from build123d import *

# Parameters (mm, degrees)
PAD_DEPTH       = 10
SKETCH001_W     = 15
SKETCH001_H     = 3
PAD001_DEPTH    = 44
SKETCH002_R     = 14
SKETCH002_R_2   = 1.7
POCKET_DEPTH    = 6.001
SKETCH003_R     = 1.2
POCKET001_DEPTH = 5
POCKET002_DEPTH = 2.5


with BuildPart() as part:
    # Sketch → Pad (new body)
    with BuildSketch(Plane.XZ):
        with BuildLine():
            Line((0, 0), (24, 0))
            ThreePointArc((24, 0), (24.707107, 0.292893), (25, 1))
            Line((25, 1), (25, 2))
            ThreePointArc((26, 3), (25.292893, 2.707107), (25, 2))
            Line((26, 3), (37, 3))
            Line((37, 3), (37, 6))
            Line((37, 6), (22, 6))
            Line((22, 6), (22, 5))
            ThreePointArc((21, 4), (21.707107, 4.292893), (22, 5))
            Line((21, 4), (0, 4))
            Line((0, 4), (0, 0))
        make_face()
    extrude(amount=PAD_DEPTH)

    # Sketch001 (on Face13 of Pad) → Pad001 (join)
    with BuildSketch(Plane.XZ.offset(10)):
        with Locations((29.5, 4.5)):
            Rectangle(SKETCH001_W, SKETCH001_H)
    extrude(amount=PAD001_DEPTH)

    # Sketch002 (on Face14 of Pad001) → Pocket (cut, through all)
    with BuildSketch(Plane(origin=(0, 0, 6), x_dir=(-1, 0, 0), z_dir=(0, 0, 1))):
        with Locations((-48, 33)):
            Circle(SKETCH002_R)
        with Locations((-32.5, 48.5)):
            Circle(SKETCH002_R_2)
        with Locations((-32.5, 17.5)):
            Circle(SKETCH002_R_2)
    extrude(amount=-POCKET_DEPTH, mode=Mode.SUBTRACT)

    # Sketch003 (on Face1 of Pocket) → Pocket001 (cut)
    with BuildSketch(Plane(origin=(0, 0, 4), x_dir=(-1, 0, 0), z_dir=(0, 0, 1))):
        with Locations((-3, 5)):
            Circle(SKETCH003_R)
        with Locations((-13, 5)):
            Circle(SKETCH003_R)
    extrude(amount=-POCKET001_DEPTH, mode=Mode.SUBTRACT)

    # Sketch004 (on Face9 of Pocket001) → Pocket002 (cut)
    with BuildSketch(Plane(origin=(0, 0, 0), x_dir=(1, 0, 0), z_dir=(0, 0, -1))):
        Polygon((4.948557, 3.875), (4.948557, 6.125), (3, 7.25), (1.051443, 6.125), (1.051443, 3.875), (3, 2.75), align=None)
        Polygon((13, 2.75), (14.948557, 3.875), (14.948557, 6.125), (13, 7.25), (11.051443, 6.125), (11.051443, 3.875), align=None)
    extrude(amount=-POCKET002_DEPTH, mode=Mode.SUBTRACT)


solid = part.part
Geometry check sheet. Reference: the model listing, model coordinates, mm. A direction names the side the tool comes from. Round coordinates to 2 decimals unless told otherwise and drop trailing zeros. Order: outer loops, then holes, each group sorted by start corner. A loop starts at its lowest first (then second) coordinate and runs counter-clockwise, first axis right, second up. Notation, with made-up numbers: M -26,35 L 12,35 A26 ccw 12,62 Z; hole C 46,-5 d10. An arc over 180 degrees is marked long. Answer in a Markdown table with one row per item. Add a question column.
Item 1: Material ranges on L1, parallel to X at y = -5, z = 3.75; L2, parallel to Y at x = 13, z = 3.2; L3, parallel to Y at x = 32.5, z = 4.55, recorded low to high. Write a range as [from, to].
Item 2: Set-up check for faces 4 (the face through (24.699, -4.93, 0.285)), 5 (the face through (1.051, -5, 1)), 6 (the face through (11, -5, 4)), 7 (the face through (30.93, -47.85, 4.52)), 8 (the face through (29, -27, 3)): record each of +Z, -Z, +X, -X, +Y, -Y from which the full face is reachable in a straight line by a thin tool's end or side.
Item 3: Sectioned sample at D-D, the plane y = -42.5. Enter the section's corners in (x, z).
Item 4: Sectioned sample at B-B, the plane y = -17.5. Enter the section's corners in (x, z), plus the area to 3 significant figures.
Item 5: Depth check by flat-ended pin: pin 1 Ø2.5 at (y, z) = (-4.5, 1) entering from +X; pin 2 Ø4 at (x, y) = (3, -5) entering from +Z; pin 3 Ø3 at (x, y) = (32.5, -48.5) entering from +Z; pin 4 Ø1.5 at (x, z) = (11, 3.5) entering from -Y. Enter the tip coordinate at first touch or a pass-through.
Item 6: Sectioned sample at A-A, the plane y = -5. Enter the section's corners in (x, z).
Item 7: Draft check along Y on faces 1 (the face through (12, -3, 0)), 2 (the face through (12.01, -3.32, 1.23)), 3 (the face through (18, 0, 3)). Enter one of: released by +Y, released by -Y, zero draft, split by the parting line, or undercut.
Item 8: Sectioned sample at C-C, the plane x = 10.5. Enter the section's corners in (y, z), plus the area to 3 significant figures.
Filled in:
| question | item | result |
|---|---|---|
| 1 | L1 | x = [0, 1.8], [4.2, 11.8], [14.2, 37] |
| 1 | L2 | y = [-10, -6.2], [-3.8, 0] |
| 1 | L3 | y = [-54, -50.2], [-46.8, -19.2], [-15.8, 0] |
| 2 | face 4 | -Z, +X, +Y, -Y |
| 2 | face 5 | -Z |
| 2 | face 6 | +Z, -X, +Y, -Y |
| 2 | face 7 | +Z, -Z |
| 2 | face 8 | -Z, +X, -Y |
| 3 | outline | M 22,3 L 37,3 L 37,6 L 22,6 Z |
| 4 | outline | M 22,3 L 30.8,3 L 30.8,6 L 22,6 Z; M 34.2,3 L 37,3 L 37,6 L 34.2,6 Z |
| 4 | area | 34.8 mm² |
| 5 | pin 1 | stops at x = 25.03 |
| 5 | pin 2 | stops at z = 4 |
| 5 | pin 3 | passes through |
| 5 | pin 4 | stops at y = -10 |
| 6 | outline | M 0,0 L 1.05,0 L 1.05,2.5 L 1.8,2.5 L 1.8,4 L 0,4 Z; M 4.2,2.5 L 4.95,2.5 L 4.95,0 L 11.05,0 L 11.05,2.5 L 11.8,2.5 L 11.8,4 L 4.2,4 Z; M 14.2,2.5 L 14.95,2.5 L 14.95,0 L 24,0 A1 ccw 25,1 L 25,2 A1 cw 26,3 L 37,3 L 37,6 L 22,6 L 22,5 A1 cw 21,4 L 14.2,4 Z |
| 7 | face 1 | zero draft |
| 7 | face 2 | undercut |
| 7 | face 3 | released by +Y |
| 8 | outline | M -10,0 L 0,0 L 0,4 L -10,4 Z |
| 8 | area | 40.0 mm² |
